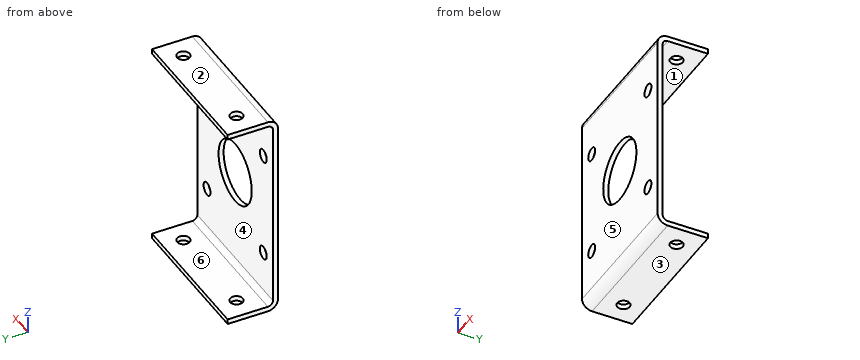
from build123d import *

# Parameters (mm, degrees)
SKETCH1_W                    = 36.195
SKETCH1_H                    = 50.038
SKETCH1_R                    = 7.9375
BASE_FLANGE1_DEPTH           = 1.27
EDGE_FLANGE1_STRIP_W         = 7.62
EDGE_FLANGE1_STRIP_H         = 1.27
EDGE_FLANGE1_STRIP_CUT_DEPTH = 36.195
EDGE_FLANGE1_DEPTH           = 36.195
SKETCH9_R                    = 1.651
CUT_EXTRUDE1_DEPTH           = 34.900972364
CUT_EXTRUDE2_DEPTH           = 57.768041099
CUT_EXTRUDE2_DEPTH_BACK      = 57.768041099
SKETCH10_R                   = 1.5875
CIRPATTERN2_COUNT            = 4


# Sheet-metal steps are written as plain solids
with BuildPart() as part:
    # Sketch1 → Base-Flange1 (new body)
    with BuildSketch(Plane(origin=(0, 0, 0), x_dir=(1, 0, 0), z_dir=(0, 1, 0))):
        Rectangle(SKETCH1_W, SKETCH1_H)
        with Locations(Location((0, 0, 0), (0, 0, 270))):
            Circle(SKETCH1_R, mode=Mode.SUBTRACT)
    extrude(amount=-BASE_FLANGE1_DEPTH)

    # Edge-Flange1 strip (across the edge) → Edge-Flange1 strip cut (cut)
    with BuildSketch(Plane(origin=(-18.0975, 0, 25.019), x_dir=(0, 0, -1), z_dir=(1, 0, 0))):
        with Locations((-2.54, -0.635)):
            Rectangle(EDGE_FLANGE1_STRIP_W, EDGE_FLANGE1_STRIP_H)
    edge_flange1_strip_cut = extrude(amount=EDGE_FLANGE1_STRIP_CUT_DEPTH, mode=Mode.SUBTRACT)

    # Edge-Flange1 section (across the edge) → Edge-Flange1 (add)
    with BuildSketch(Plane(origin=(-18.0975, 0, 25.019), x_dir=(0, 0, -1), z_dir=(1, 0, 0))):
        with BuildLine():
            Line((-1.27, 1.27), (-1.27, 11.43))
            Line((-1.27, 11.43), (0, 11.43))
            Line((0, 11.43), (0, 1.27))
            ThreePointArc((0, 1.27), (0.371974388, 0.371974388), (1.27, 0))
            Line((1.27, 0), (1.27, -1.27))
            ThreePointArc((1.27, -1.27), (-0.526051224, -0.526051224), (-1.27, 1.27))
        make_face()
    edge_flange1 = extrude(amount=EDGE_FLANGE1_DEPTH)

    # Mirror1: Edge-Flange1 strip cut, Edge-Flange1 across plane
    add(edge_flange1_strip_cut.mirror(Plane.XY), mode=Mode.SUBTRACT)
    add(edge_flange1.mirror(Plane.XY))

    # Sketch9 → Cut-Extrude1 (cut, through all)
    with BuildSketch(Plane(origin=(0, 0, 0), x_dir=(1, 0, 0), z_dir=(0, 1, 0))):
        with Locations(Location((13.462, 13.462, 0), (0, 0, 270))):
            Circle(SKETCH9_R)
    cut_extrude1 = extrude(amount=-CUT_EXTRUDE1_DEPTH, mode=Mode.SUBTRACT)

    # Sketch10 → Cut-Extrude2 (cut, two sides: drawn at the far end of the back side and taken through both)
    with BuildSketch(Plane(origin=(0, 0, -26.289), x_dir=(-1, 0, 0), z_dir=(0, 0, -1)).offset(-CUT_EXTRUDE2_DEPTH_BACK)):
        with Locations((-12.7, 6.35)):
            Circle(SKETCH10_R)
        with Locations((12.7, 6.35)):
            Circle(SKETCH10_R)
    extrude(amount=CUT_EXTRUDE2_DEPTH + CUT_EXTRUDE2_DEPTH_BACK, mode=Mode.SUBTRACT)

    # CirPattern2: Cut-Extrude1 ×4 about axis
    cirpattern2_axis = Axis((0, 0, 0), (0, 1, 0))
    for i in range(1, CIRPATTERN2_COUNT):
        add(cut_extrude1.rotate(cirpattern2_axis, i * 360 / CIRPATTERN2_COUNT), mode=Mode.SUBTRACT)


solid = part.part
The listing builds one solid part. Answer for the finished solid, in the listing's coordinates (mm). Face numbers are marked on the shaded views. A direction names the side the tool comes from. Round coordinates to 2 decimals unless told otherwise and drop trailing zeros. Write each loop counter-clockwise with the first axis right and the second up, starting at its lowest first coordinate (ties: lowest second). Pieces come first, ordered by that corner, then holes. Notation, with made-up numbers: M -23,11.5 L 9,11.5 A22 ccw 9,23.5 Z; hole C 22,51.25 d3. An arc over 180 degrees is marked long. Write each question's results on one line, items separated by ' | '. Start each with the question number.
Item 1: Find section D-D on x = 6. Write down the section's boundary in (y, z), and give its area (3 significant figures).
Item 2: Find section C-C on y = 4. Write down the section's boundary in (x, z), and give its area (3 significant figures).
Item 3: Straight lines are drawn through the part: probe 1 along X at (y, z) = (6.35, -25.45); probe 2 along Z at (x, y) = (-16, 6); probe 3 along Y at (x, z) = (0.5, 15.5). For each, find the intervals that lie inside material, in ascending order.
Item 4: The mould has two halves that part along Z. Classify the marked faces 3, 4, 5 and 6: +Z half, -Z half, draft (parallel to the pull), parting line (faces both ways), or undercut.
Item 5: Which of the six approach directions +Z, -Z, +X, -X, +Y, -Y give full straight-line access (tool end or side, diameter ignored) to the marked faces 1 and 2?
Item 6: Given pin 1 Ø12 at (x, z) = (-7, -6.5) entering from +Y, flat-ended and moving along its own axis, determine where the tip first touches the part or whether it passes through.
Item 7: Find section B-B on y = 6.35. Write down the section's boundary in (x, z).
Item 8: Find section A-A on z = 0. Write down the section's boundary in (x, y), and give its area (3 significant figures).
Answer block:
1) outline: M -1.27,-23.75 A2.54 ccw 1.27,-26.29 L 11.43,-26.29 L 11.43,-25.02 L 1.27,-25.02 A1.27 cw 0,-23.75 L 0,-5.2 L -1.27,-5.2 Z; M -1.27,5.2 L 0,5.2 L 0,23.75 A1.27 cw 1.27,25.02 L 11.43,25.02 L 11.43,26.29 L 1.27,26.29 A2.54 ccw -1.27,23.75 Z | area: 80.5 mm²
2) outline: M -18.1,-26.29 L 18.1,-26.29 L 18.1,-25.02 L -18.1,-25.02 Z; M -18.1,25.02 L 18.1,25.02 L 18.1,26.29 L -18.1,26.29 Z | area: 91.9 mm²
3) probe 1: x = -18.1 to -14.29, -11.11 to 11.11, 14.29 to 18.1 | probe 2: z = -26.29 to -25.02, 25.02 to 26.29 | probe 3: y = -1.27 to 0
4) face 3: -Z half | face 4: undercut | face 5: draft | face 6: undercut
5) face 1: +X, -X, +Y | face 2: +Z, +X, -X, +Y, -Y
6) pin 1: stops at y = 0
7) outline: M -18.1,-26.29 L -14.29,-26.29 L -14.29,-25.02 L -18.1,-25.02 Z; M -18.1,25.02 L -14.29,25.02 L -14.29,26.29 L -18.1,26.29 Z; M -11.11,-26.29 L 11.11,-26.29 L 11.11,-25.02 L -11.11,-25.02 Z; M -11.11,25.02 L 11.11,25.02 L 11.11,26.29 L -11.11,26.29 Z; M 14.29,-26.29 L 18.1,-26.29 L 18.1,-25.02 L 14.29,-25.02 Z; M 14.29,25.02 L 18.1,25.02 L 18.1,26.29 L 14.29,26.29 Z
8) outline: M -18.1,-1.27 L -7.94,-1.27 L -7.94,0 L -18.1,0 Z; M 7.94,-1.27 L 18.1,-1.27 L 18.1,0 L 7.94,0 Z | area: 25.8 mm²
